Verification items for the finished model (mm, model axes). Face numbers are marked on the shaded views. A direction names the side the tool comes from. Round coordinates to 2 decimals unless told otherwise and drop trailing zeros. Write each loop counter-clockwise with the first axis right and the second up, starting at its lowest first coordinate (ties: lowest second). Pieces come first, ordered by that corner, then holes. Notation, with made-up numbers: (-15, 5.5) - (-4, 5.5) arc R7 ccw to (-4, 10.5) - close; hole circle Ø9 at (-18, -2). An arc over 180 degrees is marked (long way). Answer as a JSON object with one key per item and string values.
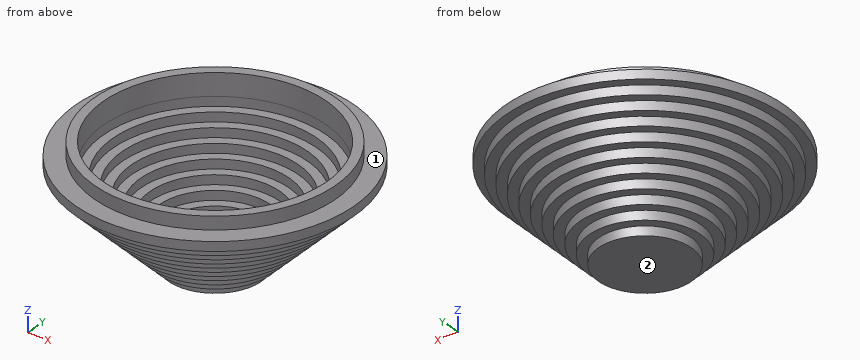
```python
from build123d import *

# Parameters (mm, degrees)
F2_R     = 130
F2_R_2   = 120
F3_DEPTH = 24


with BuildPart() as f1:
    # F0 (on Front) → F1 (revolve)
    with BuildSketch(Plane.XZ):
        Polygon((0, 10), (0, 0), (50, 0), (50, 10), (60, 10), (60, 20), (70, 20), (70, 30), (80, 30), (80, 40), (90, 40), (90, 50), (100, 50), (100, 60), (110, 60), (110, 70), (120, 70), (120, 80), (130, 80), (130, 90), (140, 90), (140, 100), (150, 100), (150, 110), (130, 110), (130, 100), (120, 100), (120, 90), (110, 90), (110, 80), (100, 80), (100, 70), (90, 70), (90, 60), (80, 60), (80, 50), (70, 50), (70, 40), (60, 40), (60, 30), (50, 30), (50, 20), (40, 20), (40, 10), align=None)
    revolve(axis=Axis((0, 0, 5), (0, 0, -1)))

    # F2 (on face) → F3 (join)
    with BuildSketch(Plane.XY.offset(100)):
        Circle(F2_R)
        Circle(F2_R_2, mode=Mode.SUBTRACT)
    extrude(amount=F3_DEPTH)


solid = f1.part
```
Q1. Material ranges on line 1 along Y through (x, z) = (0, 45.5); line 2 along Y through (x, z) = (0, 83.5); line 3 along X through (y, z) = (0, 24.75), recorded low to high. Write a range as [from, to].
Geometry check:
{"line 1": "y = [-90, -70], [70, 90]", "line 2": "y = [-130, -110], [110, 130]", "line 3": "x = [-70, -50], [50, 70]"}
Q2. Gauge pin test, flat ends, axial feed: P1, Ø4, axis at y = -97.5, z = 84, coming from the +X side; P2, Ø1.5, axis at x = 23, y = 73.5, coming from the -Z side; P3, Ø1, axis at y = -62, z = 24, coming from the -X side. Record the tip position at first contact, or that the pin passes through.
Geometry check:
{"P1": "stops at x = 88.2", "P2": "stops at z = 30", "P3": "stops at x = -33.43"}
Q3. Set-up check for the marked faces 1 and 2: record each of +Z, -Z, +X, -X, +Y, -Y from which the full face is reachable in a straight line by a thin tool's end or side.
Geometry check:
{"face 1": "+Z", "face 2": "-Z, +X, -X, +Y, -Y"}
Q4. Section check A-A, the plane y = -125. Record the cut outline in (x, z), then the cut area to 3 significant figures.
Geometry check:
{"outline": "(-82.92, 100) - (-63.05, 100) - (-63.05, 90) - (-35.71, 90) - (-35.71, 80) - (35.71, 80) - (35.71, 90) - (63.05, 90) - (63.05, 100) - (82.92, 100) - (82.92, 110) - (35.71, 110) - (35.71, 124) - (-35.71, 124) - (-35.71, 110) - (-82.92, 110) - close", "area": "4,630 mm2"}
